```python
from build123d import *

# Parameters (mm, degrees)
SKETCH1_R           = 15.875
SKETCH1_R_2         = 7.14375
SKETCH1_R_3         = 13.096875
BOSS_EXTRUDE1_DEPTH = 15.875
FILLET3_R           = 3.175
FILLET3_2_R         = 2.54


with BuildPart() as part:
    # Sketch1 → Boss-Extrude1 (new body)
    with BuildSketch(Plane(origin=(0, 0, 0), x_dir=(1, 0, 0), z_dir=(0, 1, 0))):
        with Locations((0, -45.24375)):
            Circle(SKETCH1_R)
        with Locations((0, -45.24375)):
            Circle(SKETCH1_R_2, mode=Mode.SUBTRACT)
        with BuildLine():
            ThreePointArc((15.875, 45.24375), (-1.680494891, 29.457947457), (-15.519212525, 48.585855263))
            Line((-15.519212525, 48.585855263), (-24.830740041, 5.347368421))
            ThreePointArc((-24.830740041, 5.347368421), (-25.4, 0), (-24.830740041, -5.347368421))
            Line((-24.830740041, -5.347368421), (-15.519212525, -48.585855263))
            ThreePointArc((-15.519212525, -48.585855263), (-1.680494891, -29.457947457), (15.875, -45.24375))
            ThreePointArc((15.875, -45.24375), (15.785802543, -46.924244891), (15.519212525, -48.585855263))
            Line((15.519212525, -48.585855263), (24.830740041, -5.347368421))
            ThreePointArc((24.830740041, -5.347368421), (25.4, 0), (24.830740041, 5.347368421))
            Line((24.830740041, 5.347368421), (15.519212525, 48.585855263))
            ThreePointArc((15.519212525, 48.585855263), (15.785802543, 46.924244891), (15.875, 45.24375))
        make_face()
        Circle(SKETCH1_R_3, mode=Mode.SUBTRACT)
        with Locations((0, 45.24375)):
            Circle(SKETCH1_R)
        with Locations((0, 45.24375)):
            Circle(SKETCH1_R_2, mode=Mode.SUBTRACT)
    extrude(amount=BOSS_EXTRUDE1_DEPTH)

    # Sketch2 → Revolve1 (revolve)
    with BuildSketch(Plane.XY):
        Polygon((13.096875, 31.75), (19.446875, 38.1), (19.446875, -3.175), (13.096875, -3.175), align=None)
    revolve(axis=Axis((0, -3.175, 0), (0, 1, 0)))

    # Fillet3
    fillet3_edges = [part.edges().sort_by_distance(p)[0] for p in [
        (20.174976283, 0, 26.966611842),
        (25.4, 15.875, 0),
    ]]
    fillet(fillet3_edges, radius=FILLET3_R)

    # Fillet3 2
    fillet3_2_edges = [part.edges().sort_by_distance(p)[0] for p in [
        (-19.446875, 0, 0),
    ]]
    fillet(fillet3_2_edges, radius=FILLET3_2_R)


solid = part.part
```
Build history of the part. All positions in model axes, mm. A direction names the side the tool comes from. Round coordinates to 2 decimals unless told otherwise and drop trailing zeros. Write each loop counter-clockwise with the first axis right and the second up, starting at its lowest first coordinate (ties: lowest second). Pieces come first, ordered by that corner, then holes. Notation, with made-up numbers: (-8, 77) - (34, 77) arc R25 ccw to (34, 111) - close; hole circle Ø1 at (19, -38). An arc over 180 degrees is marked (long way). Answer as CSV lines item,"result".
Q1. Drill centre lines: probe 1 along Z at (x, y) = (0, 11); probe 2 along Z at (x, y) = (-6, 15); probe 3 along X at (y, z) = (7.5, 0). Where is each one in solid material? Low to high. Write a range as [from, to].
Report:
probe 1,"z = [-61.12, -52.39], [-38.1, -13.1], [13.1, 38.1], [52.39, 61.12]"
probe 2,"z = [-58.87, -49.12], [-41.37, -11.64], [11.64, 41.37], [49.12, 58.87]"
probe 3,"x = [-25.4, -13.1], [13.1, 25.4]"
Q2. Tool access for faces 1 (the cylindrical face through (-15.432, 26.832, 11.833)), 2 (the cylindrical face through (-2.839, 14.532, 12.785)), 3 (the cylindrical face through (-15.432, -2.862, 11.833)): list every direction of +Z, -Z, +X, -X, +Y, -Y with a clear straight run to the whole face (end or side of a thin tool).
Report:
face 1,"+Y"
face 2,"+Y, -Y"
face 3,"-Y"
Q3. Cut at C-C (y = 30). Write the cut outline in (x, z).
Report:
outline,"circle Ø38.89 at (0, 0); hole circle Ø26.19 at (0, 0)"
Q4. Drop flat-ended pins along their axis: pin 1 (12 mm diameter, centred on x = 10.5, z = -6, fed in from +Y); pin 2 (4 mm diameter, centred on x = 8.5, z = -30, fed in from +Y) (3 decimals); pin 3 (12 mm diameter, centred on x = -11.5, y = 7.5, fed in from -Z); pin 4 (8.5 mm diameter, centred on x = 0, z = -45.24, fed in from +Y). Give the stop position or say it passes through.
Report:
pin 1,"stops at y = 36.75"
pin 2,"stops at y = 15.875"
pin 3,"stops at z = -60.14"
pin 4,"passes through"
Q5. Cut at B-B (z = 0). Write the cut outline in (x, y) (3 decimals), and give its area (3 significant figures).
Report:
outline,"(-25.4, 3.175) arc R3.175 ccw to (-22.225, 0) - (-21.987, 0) arc R2.54 cw to (-19.447, -2.54) - (-19.447, -3.175) - (-13.097, -3.175) - (-13.097, 31.75) - (-19.447, 38.1) - (-19.447, 15.875) - (-22.225, 15.875) arc R3.175 ccw to (-25.4, 12.7) - close; (13.097, -3.175) - (19.447, -3.175) - (19.447, -2.54) arc R2.54 cw to (21.987, 0) - (22.225, 0) arc R3.175 ccw to (25.4, 3.175) - (25.4, 12.7) arc R3.175 ccw to (22.225, 15.875) - (19.447, 15.875) - (19.447, 38.1) - (13.097, 31.75) - close"
area,"667 mm^2"
Q6. Pull direction Z, two halves, no side cores. Call faces 4 (the cylindrical face through (-0.93, 7.83, 38.16)), 5 (the cylindrical face through (-0.302, 7.871, 61.116)), 6 (the cylindrical face through (19.176, 14.97, -27.068)): +Z half, -Z half, draft (parallel to the pull), parting line (faces both ways), or undercut.
Report:
face 4,"undercut"
face 5,"+Z half"
face 6,"-Z half"
Q7. Cut at A-A (x = 0). State how many separate pieces and enclosed holes the cut face has, and give its area (3 significant figures).
Report:
separate pieces,"4"
enclosed holes,"0"
area,"1,350 mm^2"
